Design review of the part built by this model. Coordinates are the model's own, in mm. Coordinates: 2 decimals unless noted, no trailing zeros.
Q1. Clearance check with flat-ended pins moving along their axes: pin 1 Ø1.6 at (y, z) = (2, 1.5) entering from -X; pin 2 Ø1 at (y, z) = (4, 2.5) entering from +X; pin 3 Ø5 at (x, y) = (6.35, 166.69) entering from -Z. State where each tip first meets the part, or that it passes through.
Q2. The part is to be moulded in two halves that separate along Y. For faces 1 (the face through (219.79, 167.71, 1.61)), 2 (the face through (6.927, 169.287, 1.61)), 3 (the face through (113, 88, 0)), say which applies: +Y half, -Y half, draft (parallel to the pull), parting line (faces both ways), or undercut.
Q3. To check wall thickness, follow probe 1 along Y at (x, z) = (222.25, 2.3) (1 decimal); probe 2 along Y at (x, z) = (50.8, 2.05); probe 3 along X at (y, z) = (15, 0.8). State the ranges of each line that lie inside material, in increasing order.
Q4. Add section A-A, the plane z = 1.3. Give the number of separate pieces and of enclosed holes in the cut face, plus the area to 3 significant figures.
from build123d import *

# Parameters (mm, degrees)
F1_DEPTH = 3.175
F2_D     = 3.8395348837
F3_D     = 5.3258064516
F4_R     = 3.175


with BuildPart() as f1:
    # F0 (on Top) → F1 (new body)
    with BuildSketch(Plane.XY):
        with BuildLine():
            Line((12.7, 9.525), (12.7, 0))
            Line((12.7, 0), (20.6375, 0))
            Line((20.6375, 0), (20.6375, 19.05))
            Line((20.6375, 19.05), (36.5125, 19.05))
            Line((36.5125, 19.05), (36.5125, 0))
            Line((36.5125, 0), (215.9, 0))
            Line((215.9, 0), (215.9, 9.525))
            Line((215.9, 9.525), (228.6, 9.525))
            Line((228.6, 9.525), (228.6, 127))
            Line((228.6, 127), (222.25, 127))
            ThreePointArc((222.25, 127), (217.4875, 131.7625), (222.25, 136.525))
            Line((222.25, 136.525), (228.6, 136.525))
            Line((228.6, 136.525), (228.6, 173.0375))
            Line((228.6, 173.0375), (0, 173.0375))
            Line((0, 173.0375), (0, 136.525))
            Line((0, 136.525), (6.35, 136.525))
            ThreePointArc((6.35, 136.525), (11.1125, 131.7625), (6.35, 127))
            Line((6.35, 127), (0, 127))
            Line((0, 127), (0, 9.525))
            Line((0, 9.525), (12.7, 9.525))
        make_face()
    extrude(amount=F1_DEPTH)

    # F2 (through all)
    with Locations(Plane(origin=(0, 0, 0), x_dir=(1, 0, 0), z_dir=(0, 0, -1))):
        with Locations((50.8, -4.7625), (177.8, -4.7625)):
            Hole(F2_D / 2)

    # F3 (through all)
    with Locations(Plane(origin=(0, 0, 0), x_dir=(1, 0, 0), z_dir=(0, 0, -1))):
        with Locations((6.35, -166.6875), (222.25, -166.6875)):
            Hole(F3_D / 2)

    # F4
    f4_edges = [f1.edges().sort_by_distance(p)[0] for p in [
        (215.9, 9.525, 1.5875),
        (12.7, 9.525, 1.5875),
        (36.5125, 19.05, 1.5875),
        (20.6375, 19.05, 1.5875),
    ]]
    fillet(f4_edges, radius=F4_R)


solid = f1.part
Here are the results:
1. pin 1: stops at x = 12.7
1. pin 2: stops at x = 215.9
1. pin 3: passes through
2. face 1: undercut
2. face 2: undercut
2. face 3: draft
3. probe 1: y = 9.5 to 127, 136.5 to 164, 169.4 to 173
3. probe 2: y = 0 to 2.84, 6.68 to 173.04
3. probe 3: x = 0 to 20.64, 36.51 to 228.6
4. separate pieces: 1
4. enclosed holes: 4
4. area: 38,800 mm2
